For this review, use the dimensioned drawing (mm, ordinates from the lowest corner) and the shaded views. Give positions to 0.01 mm unless a question says otherwise; leave off trailing zeros. Order: outer loops, then holes, each group sorted by start corner. A loop starts at its lowest first (then second) coordinate and runs counter-clockwise, first axis right, second up. Notation, with made-up numbers: (13, 42) - (51, 42) arc R13 ccw to (51, 57) - close; hole circle Ø7 at (28.25, -3). An arc over 180 degrees is marked (long way). One line per item, written item: value.
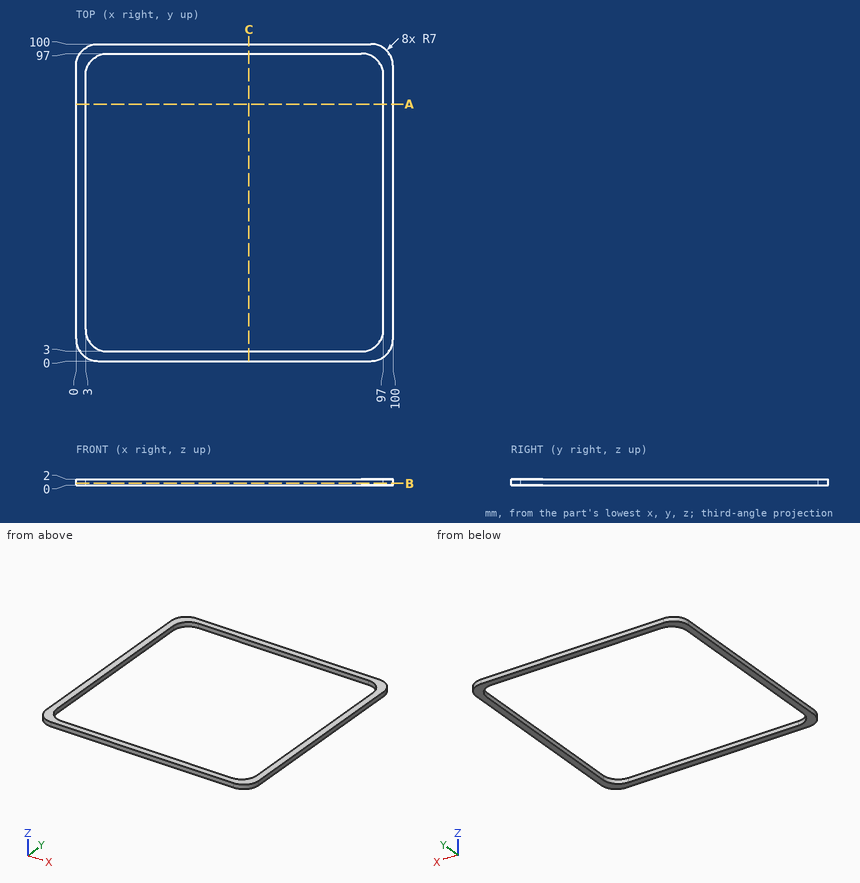
(1) Take a section at B-B (z = 0.65). Write out the cut boundary in (x, y).
Answers below:
outline: (0, 7) arc R7 ccw to (7, 0) - (93, 0) arc R7 ccw to (100, 7) - (100, 93) arc R7 ccw to (93, 100) - (7, 100) arc R7 ccw to (0, 93) - close; hole (3, 10) arc R7 ccw to (10, 3) - (90, 3) arc R7 ccw to (97, 10) - (97, 90) arc R7 ccw to (90, 97) - (10, 97) arc R7 ccw to (3, 90) - close
(2) Take a section at A-A (y = 81). Write out the cut boundary in (x, z).
Answers below:
outline: (0, 0) - (3, 0) - (3, 2) - (0, 2) - close; (97, 0) - (100, 0) - (100, 2) - (97, 2) - close
(3) Wall thickness on line 1 (X direction, y = 27.5, z = 0.4); line 2 (Y direction, x = 93, z = 1.3): over which ranges is each line inside the solid? List them lowest first. Write a range as from..to.
Answers below:
line 1: x = 0..3, 97..100
line 2: y = 0..3.68, 96.32..100
(4) For P1, Ø0.6, axis at x = 69, z = 1, coming from the -Y side, flat-tipped, find the tip position at first contact; note if it passes through.
Answers below:
P1: stops at y = 0
